Work out the finished part from the listing and answer in its coordinate system (mm). A direction names the side the tool comes from. Round coordinates to 2 decimals unless told otherwise and drop trailing zeros. Order: outer loops, then holes, each group sorted by start corner. A loop starts at its lowest first (then second) coordinate and runs counter-clockwise, first axis right, second up. Notation, with made-up numbers: M -20.75,76 L 3.25,76 A22 ccw 3.25,113 Z; hole C 48.5,79.5 d3. An arc over 180 degrees is marked long. Answer as a JSON object with one key per item and string values. Group by question number.
from build123d import *

# Parameters (mm, degrees)
SKETCH_1_W          = 15
SKETCH_1_H          = 15
SKETCH_1_W_2        = 12
SKETCH_1_H_2        = 12
EXTRUDE_1_DEPTH     = 595
CUT_EXTRUDE_2_REACH = 597.378
SKETCH_3_R          = 2.15
SKETCH_4_R          = 2.15
CUT_EXTRUDE_3_DEPTH = 596.37803117


with BuildPart() as part:
    # ｽｹｯﾁ1 → 押し出し-薄板1 (new body)
    with BuildSketch(Plane(origin=(0, 0, 0), x_dir=(1, 0, 0), z_dir=(0, 1, 0))):
        with Locations((7.5, 7.5)):
            Rectangle(SKETCH_1_W, SKETCH_1_H)
        with Locations((7.5, 7.5)):
            Rectangle(SKETCH_1_W_2, SKETCH_1_H_2, mode=Mode.SUBTRACT)
    extrude(amount=EXTRUDE_1_DEPTH)

    # ｶｯﾄ - 押し出し2: up to this face of the body (flat: up to its plane)
    cut_extrude_2_end = Plane(part.part.faces().sort_by_distance((7.5, 297.5, -15))[0])
    # ｽｹｯﾁ3 → ｶｯﾄ - 押し出し2 (cut, up to the picked face)
    with BuildSketch(Plane.XY, mode=Mode.PRIVATE) as cut_extrude_2_sk1:
        with Locations((7.5, 81)):
            Circle(SKETCH_3_R)
    cut_extrude_2_tool1 = split(extrude(cut_extrude_2_sk1.sketch, amount=-CUT_EXTRUDE_2_REACH, mode=Mode.PRIVATE), bisect_by=cut_extrude_2_end, keep=Keep.BOTH, mode=Mode.PRIVATE)
    # ｽｹｯﾁ3 → ｶｯﾄ - 押し出し2 (cut, up to the picked face)
    with BuildSketch(Plane.XY, mode=Mode.PRIVATE) as cut_extrude_2_sk2:
        with Locations((7.5, 111)):
            Circle(SKETCH_3_R)
    cut_extrude_2_tool2 = split(extrude(cut_extrude_2_sk2.sketch, amount=-CUT_EXTRUDE_2_REACH, mode=Mode.PRIVATE), bisect_by=cut_extrude_2_end, keep=Keep.BOTH, mode=Mode.PRIVATE)
    # ｽｹｯﾁ3 → ｶｯﾄ - 押し出し2 (cut, up to the picked face)
    with BuildSketch(Plane.XY, mode=Mode.PRIVATE) as cut_extrude_2_sk3:
        with Locations((7.5, 161)):
            Circle(SKETCH_3_R)
    cut_extrude_2_tool3 = split(extrude(cut_extrude_2_sk3.sketch, amount=-CUT_EXTRUDE_2_REACH, mode=Mode.PRIVATE), bisect_by=cut_extrude_2_end, keep=Keep.BOTH, mode=Mode.PRIVATE)
    # ｽｹｯﾁ3 → ｶｯﾄ - 押し出し2 (cut, up to the picked face)
    with BuildSketch(Plane.XY, mode=Mode.PRIVATE) as cut_extrude_2_sk4:
        with Locations((7.5, 191)):
            Circle(SKETCH_3_R)
    cut_extrude_2_tool4 = split(extrude(cut_extrude_2_sk4.sketch, amount=-CUT_EXTRUDE_2_REACH, mode=Mode.PRIVATE), bisect_by=cut_extrude_2_end, keep=Keep.BOTH, mode=Mode.PRIVATE)
    # ｽｹｯﾁ3 → ｶｯﾄ - 押し出し2 (cut, up to the picked face)
    with BuildSketch(Plane.XY, mode=Mode.PRIVATE) as cut_extrude_2_sk5:
        with Locations((7.5, 5)):
            Circle(SKETCH_3_R)
    cut_extrude_2_tool5 = split(extrude(cut_extrude_2_sk5.sketch, amount=-CUT_EXTRUDE_2_REACH, mode=Mode.PRIVATE), bisect_by=cut_extrude_2_end, keep=Keep.BOTH, mode=Mode.PRIVATE)
    # ｽｹｯﾁ3 → ｶｯﾄ - 押し出し2 (cut, up to the picked face)
    with BuildSketch(Plane.XY, mode=Mode.PRIVATE) as cut_extrude_2_sk6:
        with Locations((7.5, 35)):
            Circle(SKETCH_3_R)
    cut_extrude_2_tool6 = split(extrude(cut_extrude_2_sk6.sketch, amount=-CUT_EXTRUDE_2_REACH, mode=Mode.PRIVATE), bisect_by=cut_extrude_2_end, keep=Keep.BOTH, mode=Mode.PRIVATE)
    add(cut_extrude_2_tool1.solids().sort_by(Axis((7.5, 81, 0), (0, 0, -1)))[0], mode=Mode.SUBTRACT)
    add(cut_extrude_2_tool2.solids().sort_by(Axis((7.5, 111, 0), (0, 0, -1)))[0], mode=Mode.SUBTRACT)
    add(cut_extrude_2_tool3.solids().sort_by(Axis((7.5, 161, 0), (0, 0, -1)))[0], mode=Mode.SUBTRACT)
    add(cut_extrude_2_tool4.solids().sort_by(Axis((7.5, 191, 0), (0, 0, -1)))[0], mode=Mode.SUBTRACT)
    add(cut_extrude_2_tool5.solids().sort_by(Axis((7.5, 5, 0), (0, 0, -1)))[0], mode=Mode.SUBTRACT)
    add(cut_extrude_2_tool6.solids().sort_by(Axis((7.5, 35, 0), (0, 0, -1)))[0], mode=Mode.SUBTRACT)

    # ｽｹｯﾁ4 → ｶｯﾄ - 押し出し3 (cut, through all)
    with BuildSketch(Plane(origin=(15, 0, 0), x_dir=(-1, 0, 0), z_dir=(0, 0, -1))):
        with Locations(Location((7.5, 577.5, 0), (0, 0, 180))):
            Circle(SKETCH_4_R)
        with Locations(Location((7.5, 590, 0), (0, 0, 180))):
            Circle(SKETCH_4_R)
        with Locations(Location((7.5, 332.5, 0), (0, 0, 180))):
            Circle(SKETCH_4_R)
    extrude(amount=CUT_EXTRUDE_3_DEPTH, mode=Mode.SUBTRACT)


solid = part.part
Item 1: Find section A-A (z = -9.5). Give the vertices of the cut face in (x, y).
Item 2: The mould has two halves that part along X. Classify faces 3 (the flat face through (14, 595, -8)), 4 (the flat face through (15, 293, -7)), 5 (the flat face through (0, 293, -7)), 6 (the flat face through (13.5, 293, -7)): +X half, -X half, draft (parallel to the pull), parting line (faces both ways), or undercut.
Item 3: A tool of negligible diameter and unlimited length cuts with its end or side. For faces 1 (the flat face through (7, 293, -15)), 2 (the flat face through (7, 293, -13.5)), from which of +Z, -Z, +X, -X, +Y, -Y can it reach the whole face along a straight path? Write none if from no direction.
Item 4: Consider L1, parallel to Z at x = 9, y = 378.5; L2, parallel to X at y = 191, z = -14.7; L3, parallel to X at y = 202.5, z = -6. Determine where each line is inside the solid, lowest interval first.
Item 5: This flat-tipped pin is pushed along its axis until it touches: pin 1 (3.5 mm diameter, centred on x = 7.5, y = 191, fed in from +Z). Where does it stop, or does it pass through?
Item 6: Find section B-B (y = 425). Give the vertices of the cut face in (x, z).
Responses:
{
 "1": {"outline": "M 0,0 L 1.5,0 L 1.5,595 L 0,595 Z; M 13.5,0 L 15,0 L 15,595 L 13.5,595 Z"},
 "2": {"face 3": "draft", "face 4": "+X half", "face 5": "-X half", "face 6": "undercut"},
 "3": {"face 1": "-Z, +X, -X, +Y, -Y", "face 2": "+Y, -Y"},
 "4": {"L1": "z = -15 to -13.5, -1.5 to 0", "L2": "x = 0 to 5.35, 9.65 to 15", "L3": "x = 0 to 1.5, 13.5 to 15"},
 "5": {"pin 1": "passes through"},
 "6": {"outline": "M 0,-15 L 15,-15 L 15,0 L 0,0 Z; hole M 1.5,-13.5 L 13.5,-13.5 L 13.5,-1.5 L 1.5,-1.5 Z"}
}
